Model file for the job. Use its own axes, mm. Face numbers are marked on the shaded views. A direction names the side the tool comes from. Round coordinates to 2 decimals unless told otherwise and drop trailing zeros. Loops run counter-clockwise (first coordinate to the right, second up) from the corner with the lowest first, then second, coordinate; pieces in that order, holes last. Notation, with made-up numbers: M -15.5,-25.75 L 15.5,-25.75 A37 ccw 15.5,12.25 Z; hole C -22.5,33 d5. An arc over 180 degrees is marked long. Use a Markdown table: item, result. Add a question column.
Item 1: Wall check: L1, parallel to Y at x = 14.1, z = 8; L2, parallel to X at y = 10, z = 9.25; L3, parallel to X at y = 114.5, z = 8. Give the ranges that are in metal, low to high. Write a range as from..to.
Item 2: Pin check, flat tips, straight feed: P1, Ø5.5, axis at x = 29.5, z = 8, coming from the +Y side; P2, Ø1.5, axis at y = 63, z = 2, coming from the -X side; P3, Ø5.5, axis at x = 22.5, z = 8, coming from the -Y side. Stop position of each tip, or through.
Item 3: Two-plate mould, pull along Y, no slides. Class the marked faces 4, 5 and 6: +Y half, -Y half, draft (parallel to the pull), parting line (faces both ways), or undercut.
Item 4: Tool access for the marked faces 1, 2 and 3: list every direction of +Z, -Z, +X, -X, +Y, -Y with a clear straight run to the whole face (end or side of a thin tool).
Item 5: Saw through at B-B on z = 14.75. Write the cut outline in (x, y), then the cut area to 3 significant figures.
Item 6: Saw through at A-A on y = 85. Write the cut outline in (x, z), then the cut area to 3 significant figures.
Item 7: Saw through at C-C on z = 2.25. Write the cut outline in (x, y), then the cut area to 3 significant figures.
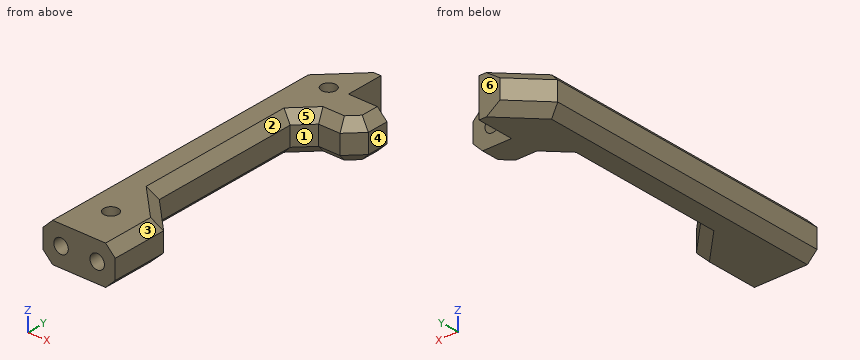
Autodesk Inventor part; units mm, degrees
ref_plane "Work Plane3" through (21.5, 121.1711, 16) normal (0, 1, 0) x (1, 0, 0)
ref_plane "Work Plane2" through (4, 0, 0) normal (0, -1, 0) x (1, 0, 0)
ref_plane "YZ Plane" through (0, 0, 0) normal (1, 0, 0) x (0, 1, 0)
sketch "Sketch1" plane through (0, 0, 0) normal (0, 0, 1) x (1, 0, 0)
  line L0 (37.5, 112.2656) -> (37.5, -3.3598) construction
  line L1 (37.5, 136.6711) -> (12.8431, 136.6711)
  line L2 (12.8431, 136.6711) -> (3.4308, 127.2588)
  line L3 (21.5, 136.6711) -> (21.5, 121.1711)
  line L4 (21.5, 121.1711) -> (37.5, 121.1711)
  line L5 (7.5005, 125.6717) -> (18.5, 136.6711) construction
  circle A0 centre (74.25, 61.25) radius 56.25 construction
  line L6 (37.5, 121.1711) -> (111, 121.1711) construction
  line L7 (111, 121.1711) -> (111, 150.3493) construction
  line L8 (111, 150.3493) -> (37.5, 150.3493) construction
  line L9 (37.5, 150.3493) -> (37.5, 121.1711) construction
  line L10 (37.5, 112.2656) -> (31.2028, 105.9683)
  line L11 (31.2028, 105.9683) -> (22.2972, 105.9683)
  line L12 (22.2972, 105.9683) -> (16, 99.6711)
  line L13 (16, 99.6711) -> (16, 37.1221)
  line L14 (16, 37.1221) -> (30, 23.1221)
  line L15 (30, 23.1221) -> (30, 0)
  line L16 (30, 0) -> (0, 0)
  line L17 (0, 0) -> (0, 123.828)
  line L18 (3.4308, 127.2588) -> (0, 123.828)
  line L19 (18, 73.8677) -> (18, 48.6323) construction
  line L20 (83.3625, 5) -> (65.1375, 5) construction
  line L21 (37.5, 121.1711) -> (37.5, 136.6711)
  line L22 (37.5, 121.1711) -> (37.5, 112.2656)
  line L23 (35.2471, 20.7034) -> (29.4259, 26.5246) construction
  point P0 (19.5296, 140.85)
  point P1 (74.25, 121.1711)
  point P2 (18, 61.25)
  point P3 (74.25, 5)
  dimension "d32" = 15.5
  dimension "d33" = 16
  dimension "d34" = 8.6569
  dimension "d38" = 4
  dimension "d39" = 3
  dimension "d65" = 112.5
  dimension "d66" = 70.293
  dimension "d67" = 73.5
  dimension "d70" = 45
  dimension "d71" = 16
  dimension "d72" = 2
  dimension "d73" = 5
  dimension "d74" = 30
  dimension "d75" = 2
extrude "Extrusion2" add sketch "Sketch1" along normal blind 16 contours L3 L4 L22 L10 L11 L12 L13 L14 L15 L16 L17 L18 L2 L1
ref_plane "Work Plane3" through (21.5, 121.1711, 16) normal (0, 1, 0) x (1, 0, 0)
sketch "Sketch4" plane through (21.5, 121.1711, 16) normal (0, 1, 0) x (1, 0, 0)
  circle A0 centre (8, 8) radius 3
  line L0 (16, 16) -> (0, 16)
  line L1 (16, 16) -> (16, 0)
  point P0 (-21.5, 16)
  point P1 (16, 8)
  point P2 (8, 16)
  dimension "d76" = 6
hole "Hole1" at (29.5, 121.1711, 8) direction (0, -1, 0) diameter 6 depth 9.5 tip angle 118
ref_plane "Work Plane2" through (4, 0, 0) normal (0, -1, 0) x (1, 0, 0)
sketch "Sketch5" plane through (4, 0, 0) normal (0, -1, 0) x (1, 0, 0)
  circle A0 centre (3.5, 8) radius 3
  line L0 (11, 48.9313) -> (11, 41.3239)
  circle A1 centre (18.5, 8) radius 3
  line L1 (-4, 0) -> (26, 0)
  line L2 (26, 0) -> (26, 16)
  point P0 (11, 0)
  point P1 (26, 8)
  dimension "d52" = 6
  dimension "d77" = 15
hole "Hole2" at (7.5, 0, 8) at (22.5, 0, 8) direction (0, 1, 0) diameter 6 depth 15 tip angle 118
thread "Thread4"
thread "Thread5"
chamfer "Chamfer2" distance 4 angle 45 18 edges at (0, 61.914, 16) (6.4216, 130.2496, 16) (6.4216, 130.2496, 0) (0, 61.914, 0) (34.3514, 109.1169, 0) (26.75, 105.9683, 0) (19.1486, 102.8197, 0) (16, 68.3966, 0) (23, 30.1221, 0) (30, 11.561, 0) (34.3514, 109.1169, 16) (26.75, 105.9683, 16) (19.1486, 102.8197, 16) (16, 68.3966, 16) (23, 30.1221, 16) (30, 11.561, 16) (37.5, 116.7183, 16) (37.5, 116.7183, 0)
sketch "Sketch6" plane through (0, 0, 16) normal (0, 0, 1) x (1, 0, 0)
  circle A0 centre (14.1, 120.25) radius 3
  circle A1 centre (14.1, 16.25) radius 3
  line L0 (4, 0) -> (4, 122.1711)
  circle A2 centre (74.25, 61.25) radius 56.25 construction
  circle A3 centre (74.25, 61.25) radius 50 construction
  line L1 (74.25, 111.25) -> (10.3895, 111.25) construction
  line L2 (0, 0) -> (4, 0)
  dimension "d88" = 100
  dimension "d85" = 6
  dimension "d86" = 10.1
  dimension "d89" = 9
  dimension "d103" = 104
hole "Hole3" at (14.1, 120.25, 16) at (14.1, 16.25, 16) direction (0, 0, -1) diameter 6 depth 10 tip angle 118
thread "Thread8"
thread "Thread9"
properties part number "rackstand-v2-left"
Entries:
| question | item | result |
|---|---|---|
| 1 | L1 | 0..13.25, 19.25..117.25, 123.25..136.67 |
| 1 | L2 | 0..4.77, 10.23..19.77, 25.23..30 |
| 1 | L3 | 0..26.5, 32.5..37.5 |
| 2 | P1 | y = 111.52 |
| 2 | P2 | x = 1.25 |
| 2 | P3 | y = 15.15 |
| 3 | face 4 | draft |
| 3 | face 5 | undercut |
| 3 | face 6 | +Y half |
| 4 | face 1 | +Z, -Z, +X |
| 4 | face 2 | +Z, +X |
| 4 | face 3 | +Z, +X, -Y |
| 5 | outline | M 2.75,0 L 27.25,0 L 27.25,21.98 L 13.25,35.98 L 13.25,100.81 L 21.16,108.72 L 30.06,108.72 L 34.75,113.4 L 34.75,121.17 L 21.5,121.17 L 21.5,136.67 L 16.73,136.67 L 2.75,122.69 Z; hole C 14.1,16.25 d6; hole C 14.1,120.25 d6 |
| 5 | area | 2,100 mm2 |
| 6 | outline | M 0,4 L 4,0 L 12,0 L 16,4 L 16,12 L 12,16 L 4,16 L 0,12 Z |
| 6 | area | 224 mm2 |
| 7 | outline | M 1.75,0 L 28.25,0 L 28.25,22.4 L 14.25,36.4 L 14.25,100.4 L 21.57,107.72 L 30.48,107.72 L 35.75,112.99 L 35.75,121.17 L 21.5,121.17 L 21.5,136.67 L 15.32,136.67 L 1.75,123.1 Z |
| 7 | area | 2,440 mm2 |
